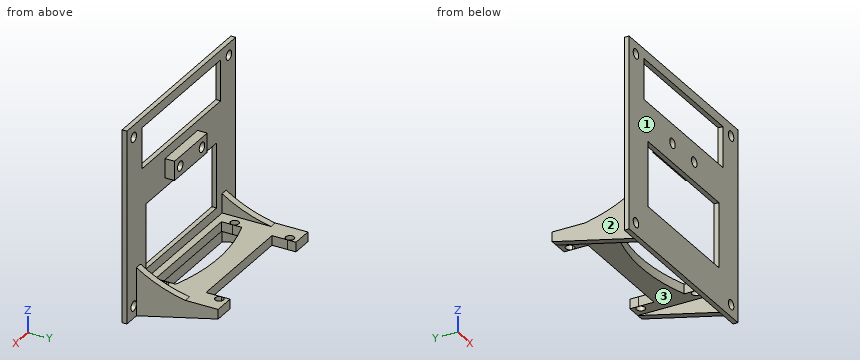
Autodesk Inventor part; units mm, degrees
ref_plane "YZ Plane" through (0, 0, 0) normal (1, 0, 0) x (0, 1, 0)
ref_plane "XZ Plane" through (0, 0, 0) normal (0, 1, 0) x (-1, 0, 0)
ref_plane "XY Plane" through (0, 0, 0) normal (0, 0, 1) x (1, 0, 0)
sketch "Sketch1" plane through (0, 0, 0) normal (0, 1, 0) x (-1, 0, 0)
  line L0 (0, 0) -> (80, 0)
  line L1 (80, 0) -> (80, -80)
  line L2 (80, -80) -> (0, -80)
  line L3 (0, -80) -> (0, 0)
  line L4 (63.0847, -18.93) -> (13.0847, -18.93) construction
  line L5 (13.0847, -18.93) -> (13.0847, -23.93) construction
  line L6 (13.0847, -23.93) -> (63.0847, -23.93) construction
  line L7 (63.0847, -23.93) -> (63.0847, -18.93) construction
  line L8 (63.0847, -42.93) -> (13.0847, -42.93) construction
  line L9 (13.0847, -42.93) -> (13.0847, -47.93) construction
  line L10 (13.0847, -47.93) -> (63.0847, -47.93) construction
  line L11 (63.0847, -47.93) -> (63.0847, -42.93) construction
  line L12 (51.4414, -53.454) -> (27.4414, -53.454) construction
  line L13 (27.4414, -53.454) -> (27.4414, -61.454) construction
  line L14 (27.4414, -61.454) -> (51.4414, -61.454) construction
  line L15 (51.4414, -61.454) -> (51.4414, -53.454) construction
  circle A0 centre (48.4614, -57.454) radius 2 construction
  circle A1 centre (30.4614, -57.454) radius 2 construction
  dimension "d0" = 80
  dimension "d1" = 80
  dimension "d2" = 24
  dimension "d3" = 8
  dimension "d4" = 4
  dimension "d5" = 18
  dimension "d6" = 2.98
  dimension "d7" = 4
  dimension "d8" = 3.02
  dimension "d9" = 50
  dimension "d10" = 5
  dimension "d11" = 19
extrude "Extrusion1" add sketch "Sketch1" along normal blind 2
sketch "Sketch3" plane through (0, 2, 0) normal (0, 1, 0) x (1, 0, 0)
  circle A0 centre (-48.98, 29) radius 2 construction
  circle A1 centre (-30.98, 29) radius 2 construction
  line L0 (-28, 33) -> (-52, 33)
  line L1 (-52, 25) -> (-28, 25)
  line L2 (-28, 25) -> (-28, 33)
  line L3 (-52, 33) -> (-52, 25)
  line L4 (-80, 80) -> (-80, 0) construction
  line L5 (-80, 40) -> (0, 40) construction
  line L6 (0, 0) -> (0, 80) construction
  line L7 (0, 80) -> (-80, 80) construction
  line L8 (-40, 80) -> (-40, 0) construction
  line L9 (-80, 0) -> (0, 0) construction
  point P0 (-40, 33)
  dimension "d29" = 24
  dimension "d30" = 8
  dimension "d31" = 4
  dimension "d32" = 18
  dimension "d33" = 2.98
  dimension "d34" = 4
  dimension "d35" = 3.02
  dimension "d128" = 15
extrude "Extrusion3" add sketch "Sketch3" along normal blind 4
sketch "Sketch4" plane through (0, 2, 0) normal (0, 1, 0) x (1, 0, 0)
  point P0 (0, 0)
sketch "Sketch7" plane through (0, 2, 0) normal (0, 1, 0) x (1, 0, 0)
  line L0 (-5, 5) -> (-75, 5)
  line L1 (-75, 5) -> (-75, 75)
  line L2 (-75, 75) -> (-5, 75)
  line L3 (-5, 75) -> (-5, 5)
  line L4 (-80, 0) -> (0, 0)
  line L5 (0, 0) -> (0, 80)
  line L6 (-80, 80) -> (-80, 0)
  line L7 (0, 80) -> (-80, 80)
  dimension "d49" = 5
  dimension "d50" = 5
  dimension "d51" = 5
  dimension "d52" = 5
hole "Hole2" at (-5, 2, -5) at (-5, 2, -75) at (-75, 2, -75) at (-75, 2, -5) direction (0, -1, 0) diameter 4 end through all
sketch "Sketch10" plane through (0, 6, 0) normal (0, 1, 0) x (1, 0, 0)
  line L0 (-52, 33) -> (-52, 25)
  line L1 (-52, 29) -> (-29.1848, 29)
  point P0 (0, 0)
  point P1 (-48.1206, 29)
  point P2 (-32.1206, 29)
  dimension "d81" = 16
hole "Hole3" at (-48.1206, 6, -29) at (-32.1206, 6, -29) direction (0, -1, 0) diameter 4 end through all
sketch "Sketch20" plane through (0, 2, 0) normal (0, 1, 0) x (1, 0, 0)
  line L0 (-73, 80) -> (-70, 80) construction
  line L1 (-70, 60) -> (-73, 60) construction
  line L2 (-73, 60) -> (-73, 80) construction
  line L3 (-10, 60) -> (-7, 60) construction
  line L4 (-7, 60) -> (-7, 80) construction
  line L5 (-7, 80) -> (-10, 80) construction
  line L6 (-70, 60) -> (-73, 60)
  line L7 (-73, 60) -> (-73, 80)
  line L8 (-73, 80) -> (-70, 80)
  line L9 (-70, 80) -> (-70, 72)
  line L10 (-70, 72) -> (-10, 72)
  line L11 (-10, 72) -> (-10, 80)
  line L12 (-10, 80) -> (-7, 80)
  line L13 (-7, 80) -> (-7, 60)
  line L14 (-7, 60) -> (-10, 60)
  line L15 (-10, 60) -> (-10, 68)
  line L16 (-10, 68) -> (-70, 68)
  line L17 (-70, 68) -> (-70, 60)
  line L18 (-70, 60) -> (-73, 60)
  point P0 (0, 0)
  dimension "d132" = 3
  dimension "d133" = 20
extrude "Extrusion13" add sketch "Sketch20" along normal blind 34
sketch "Sketch21" plane through (-70, 2, -60) normal (1, 0, 0) x (0, 0, -1)
  line L0 (8, 0) -> (0, 0) construction
  line L1 (0, 0) -> (5.8768, 9.0116) construction
  line L2 (8, 0) -> (8, 34) construction
  line L3 (5.8768, 9.0116) -> (8, 20.3813) construction
  spline S0 degree 2 poles (0, 0) (5.8768, 9.0116) (8, 20.3813) knots 1 1 1 2 2 2
  line L4 (0, 0) -> (0, 34)
  line L5 (0, 0) -> (0, 34)
  line L6 (0, 34) -> (8, 34)
  line L7 (0, 34) -> (8, 34)
  line L8 (8, 34) -> (8, 20.3813)
  point P0 (-60, -2)
extrude "Extrusion14" cut sketch "Sketch21" along normal through all both and the other way through all
sketch "Sketch22" plane through (-70, 2, -72) normal (1, 0, 0) x (0, 0, -1)
  line L0 (0, 34) -> (8, 0)
  line L1 (8, 0) -> (8, 34)
  line L2 (0, 34) -> (8, 34)
  line L3 (8, 34) -> (0, 34)
  point P0 (-72, -2)
extrude "Extrusion15" cut sketch "Sketch22" along normal through all both and the other way through all
sketch "Sketch23" plane through (-70, 2, -68) normal (0, 0, 1) x (1, 0, 0)
  line L0 (4, 7.5) -> (56, 7.5)
  line L1 (56, 7.5) -> (56, 30.5)
  line L2 (56, 30.5) -> (4, 30.5)
  line L3 (4, 30.5) -> (4, 7.5)
  line L4 (4, 7.5) -> (56, 30.5)
  line L5 (56, 7.5) -> (4, 30.5)
  line L6 (30, 30.5) -> (30, 34) construction
  line L7 (-3, 34) -> (63, 34) construction
  line L8 (30, 7.5) -> (30, 4) construction
  line L9 (18, 4) -> (42, 4)
  point P0 (70, -2)
  point P1 (30, 19)
  dimension "d142" = 52
  dimension "d143" = 23
hole "Hole5" at (-14, 32.5, -68) at (-14, 9.5, -68) at (-66, 9.5, -68) at (-66, 32.5, -68) direction (0, 0, -1) diameter 3.5 end through all
sketch "Sketch24" plane through (-70, 2, -68) normal (0, 0, 1) x (1, 0, 0)
  line L0 (60, 34) -> (0, 34) construction
  line L1 (5.75, 34) -> (54.25, 34)
  line L2 (54.25, 34) -> (54.25, 24)
  line L3 (54.25, 24) -> (5.75, 24)
  line L4 (5.75, 24) -> (5.75, 34)
  circle A0 centre (4, 30.5) radius 1.75 construction
  circle A1 centre (56, 30.5) radius 1.75 construction
  point P0 (70, -2)
  dimension "d151" = 0
  dimension "d152" = 0
  dimension "d153" = 10
extrude "Extrusion16" cut sketch "Sketch24" against normal blind 34
sketch "Sketch25" plane through (-70, 2, -68) normal (0, 0, 1) x (1, 0, 0)
  line L0 (5.75, 3) -> (54.25, 3)
  line L1 (54.25, 3) -> (54.25, 11.4232)
  line L2 (54.25, 11.4232) -> (5.75, 11.4232) construction
  line L3 (5.75, 11.4232) -> (5.75, 3)
  line L4 (60, 0) -> (0, 0) construction
  circle A0 centre (4, 7.5) radius 1.75 construction
  circle A1 centre (56, 7.5) radius 1.75 construction
  arc A2 (54.25, 11.4232) -> (5.75, 11.4232) centre (30, -60.0846) ccw
  line L5 (30, 15.4232) -> (30, 11.4232) construction
  point P0 (70, -2)
  dimension "d156" = 3
  dimension "d157" = 8.4232
  dimension "d159" = 0
  dimension "d160" = 0
  dimension "d161" = 4
extrude "Extrusion17" cut sketch "Sketch25" against normal blind 34
sketch "Sketch26" plane through (0, 2, 0) normal (0, 1, 0) x (1, 0, 0)
  line L0 (-66, 64) -> (-14, 64)
  line L1 (-14, 64) -> (-14, 37)
  line L2 (-14, 37) -> (-66, 37)
  line L3 (-66, 37) -> (-66, 64)
  line L4 (-70, 68) -> (-70, 60) construction
  line L5 (-10, 60) -> (-10, 68)
  line L6 (-15.75, 68) -> (-64.25, 68) construction
  line L7 (-28, 33) -> (-52, 33)
  line L8 (-80, 0) -> (0, 0) construction
  dimension "d164" = 4
  dimension "d165" = 4
  dimension "d166" = 4
  dimension "d167" = 4
extrude "Extrusion18" cut sketch "Sketch26" against normal blind 34
sketch "Sketch27" plane through (0, 2, 0) normal (0, 1, 0) x (1, 0, 0)
  line L0 (-69, 21) -> (-11, 21)
  line L1 (-11, 21) -> (-11, 4)
  line L2 (-11, 4) -> (-69, 4)
  line L3 (-69, 4) -> (-69, 21)
  line L4 (-52, 25) -> (-28, 25) construction
  line L5 (-80, 0) -> (0, 0) construction
  circle A0 centre (-75, 5) radius 2 construction
  circle A1 centre (-5, 5) radius 2 construction
  dimension "d172" = 4
  dimension "d173" = 4
  dimension "d174" = 4
  dimension "d175" = 4
extrude "Extrusion19" cut sketch "Sketch27" against normal blind 34
properties part number "ProtoBoard"
Here's how the part is built. I have some questions about the finished solid (model axes, mm). Face numbers are marked on the shaded views. Give positions to 0.01 mm unless a question says otherwise; leave off trailing zeros. Loops run counter-clockwise (first coordinate to the right, second up) from the corner with the lowest first, then second, coordinate; pieces in that order, holes last. Notation, with made-up numbers: (0.5, 79.25) -> (12.5, 79.25) arc R20 ccw to (12.5, 90.25) -> close; hole circle Ø1 at (34.25, 59.5). An arc over 180 degrees is marked (long way). Use one line per item in the form item = value. Start each with the question number.
1) Imagine slicing it at A-A (z = -17). Please give me the cut outline in (x, y), then the cut area to 3 significant figures.
2) Imagine slicing it at D-D (z = -5). Please give me the cut outline in (x, y).
3) Thinking about a two-plate mould opening in X: for the marked faces 1, 2 and 3, which applies, +X half, -X half, draft (parallel to the pull), parting line (faces both ways), or undercut?
4) Imagine slicing it at B-B (z = -29). Please give me the cut outline in (x, y), then the cut area to 3 significant figures.
5) Please list where these lines run through material, in increasing order: line 1 along X through (y, z) = (0.9, -75); line 2 along X through (y, z) = (1, -5); line 3 along Y through (x, z) = (-66, -70.55).
6) For P1, Ø6, axis at x = -38.5, y = 23, coming from the -Z side; P2, Ø10, axis at x = -10, z = -39.5, coming from the +Y side; P3, Ø9, axis at y = 9.5, z = -64.5, coming from the +X side, each with a flat end and sliding along its axis, tell me the tip position at first contact or that it passes through.
7) Imagine slicing it at C-C (x = -75). Please give me the cut outline in (y, z), then the cut area to 3 significant figures.
Check values:
q1.outline = (-80, 0) -> (-69, 0) -> (-69, 2) -> (-80, 2) -> close; (-11, 0) -> (0, 0) -> (0, 2) -> (-11, 2) -> close
q1.area = 44.0 mm^2
q2.outline = (-80, 0) -> (-77, 0) -> (-77, 2) -> (-80, 2) -> close; (-73, 0) -> (-69, 0) -> (-69, 2) -> (-73, 2) -> close; (-11, 0) -> (-7, 0) -> (-7, 2) -> (-11, 2) -> close; (-3, 0) -> (0, 0) -> (0, 2) -> (-3, 2) -> close
q3.face_1 = draft
q3.face_2 = -X half
q3.face_3 = undercut
q4.outline = (-80, 0) -> (-50.12, 0) -> (-50.12, 6) -> (-52, 6) -> (-52, 2) -> (-80, 2) -> close; (-46.12, 0) -> (-34.12, 0) -> (-34.12, 6) -> (-46.12, 6) -> close; (-30.12, 0) -> (0, 0) -> (0, 2) -> (-28, 2) -> (-28, 6) -> (-30.12, 6) -> close
q4.area = 208 mm^2
q5.line_1 = -80 to -77, -73 to -7, -3 to 0
q5.line_2 = -80 to -77, -73 to -69, -11 to -7, -3 to 0
q5.line_3 = 0 to 7.75, 11.25 to 30.75, 34.25 to 36
q6.P1 = -72
q6.P2 = 2
q6.P3 = -7
q7.outline = (0, -80) -> (2, -80) -> (2, -77) -> (0, -77) -> close; (0, -73) -> (2, -73) -> (2, -7) -> (0, -7) -> close; (0, -3) -> (2, -3) -> (2, 0) -> (0, 0) -> close
q7.area = 144 mm^2
